Autodesk Inventor part; units mm, degrees
ref_plane "YZ Plane" through (0, 0, 0) normal (1, 0, 0) x (0, 1, 0)
ref_plane "XZ Plane" through (0, 0, 0) normal (0, 1, 0) x (-1, 0, 0)
ref_plane "XY Plane" through (0, 0, 0) normal (0, 0, 1) x (1, 0, 0)
sketch "Sketch1" plane through (0, 0, 0) normal (0, 0, 1) x (1, 0, 0)
  line L0 (0, 0) -> (112.522, 0)
  line L1 (112.522, 0) -> (112.522, 146.812)
  line L2 (112.522, 146.812) -> (0, 146.812)
  line L3 (0, 146.812) -> (0, 0)
  line L4 (7.62, 131.572) -> (104.902, 131.572)
  line L5 (104.902, 131.572) -> (104.902, 91.44)
  line L6 (104.902, 91.44) -> (7.62, 91.44)
  line L7 (7.62, 91.44) -> (7.62, 131.572)
  line L8 (21.59, 83.82) -> (90.932, 83.82)
  line L9 (90.932, 83.82) -> (90.932, 6.35)
  line L10 (90.932, 6.35) -> (21.59, 6.35)
  line L11 (21.59, 6.35) -> (21.59, 83.82)
  dimension "d0" = 97.282
  dimension "d1" = 40.132
  dimension "d2" = 69.342
  dimension "d3" = 77.47
  dimension "d4" = 6.35
  dimension "d5" = 21.59
  dimension "d6" = 7.62
  dimension "d7" = 7.62
  dimension "d8" = 15.24
  dimension "d9" = 7.62
extrude "Extrusion1" add sketch "Sketch1" along normal blind 9.4996 contours L3 L2 L1 L0 | L8 L9 L10 L11
sketch "Sketch2" plane through (0, 0, 9.4996) normal (0, 0, 1) x (1, 0, 0)
  line L0 (0, 0) -> (112.522, 0)
  line L1 (112.522, 0) -> (112.522, 139.192)
  line L2 (112.522, 139.192) -> (0, 139.192)
  line L3 (0, 139.192) -> (0, 0)
  line L4 (7.62, 131.572) -> (104.902, 131.572)
  line L5 (104.902, 131.572) -> (104.902, 91.44)
  line L6 (104.902, 91.44) -> (7.62, 91.44)
  line L7 (7.62, 91.44) -> (7.62, 131.572)
  line L8 (21.59, 83.82) -> (90.932, 83.82)
  line L9 (90.932, 83.82) -> (90.932, 6.35)
  line L10 (90.932, 6.35) -> (21.59, 6.35)
  line L11 (21.59, 6.35) -> (21.59, 83.82)
  line L12 (20.32, 85.09) -> (92.202, 85.09)
  line L13 (92.202, 85.09) -> (92.202, 5.08)
  line L14 (92.202, 5.08) -> (20.32, 5.08)
  line L15 (20.32, 5.08) -> (20.32, 85.09)
  dimension "d12" = 97.282
  dimension "d13" = 40.132
  dimension "d14" = 69.342
  dimension "d15" = 77.47
  dimension "d16" = 6.35
  dimension "d17" = 21.59
  dimension "d18" = 7.62
  dimension "d19" = 7.62
  dimension "d20" = 7.62
  dimension "d21" = 7.62
  dimension "d33" = 1.27
  dimension "d34" = 1.27
  dimension "d35" = 1.27
  dimension "d36" = 1.27
extrude "Extrusion2" cut sketch "Sketch2" against normal blind 0.0025 contours L12 L13 L14 L15
sketch "Sketch3" plane through (0, 0, 9.4996) normal (0, 0, 1) x (1, 0, 0)
  circle A0 centre (9.7155, 138.9888) radius 1.651
  circle A1 centre (102.7811, 138.9888) radius 1.651
  circle A2 centre (102.7811, 84.0232) radius 1.651
  circle A3 centre (9.7155, 84.0232) radius 1.651
  line L0 (104.902, 131.572) -> (104.902, 91.44)
  line L1 (104.902, 91.44) -> (7.62, 91.44)
  line L2 (21.59, 6.35) -> (90.932, 6.35)
  line L3 (92.202, 5.08) -> (20.32, 5.08)
  line L4 (46.101, 6.35) -> (66.421, 6.35)
  line L5 (66.421, 6.35) -> (66.421, 5.08)
  line L6 (66.421, 5.08) -> (46.101, 5.08)
  line L7 (46.101, 5.08) -> (46.101, 6.35)
  line L8 (21.59, 83.82) -> (21.59, 6.35)
  line L9 (90.932, 6.35) -> (90.932, 83.82)
  point P0 (0, 0)
  dimension "d24" = 3.302
  dimension "d25" = 93.0656
  dimension "d26" = 93.0656
  dimension "d27" = 0
  dimension "d28" = 54.9656
  dimension "d29" = 2.1209
  dimension "d30" = 0
  dimension "d31" = 7.4168
  dimension "d32" = 0
  dimension "d37" = 20.32
  dimension "d38" = 24.511
  dimension "d39" = 24.511
extrude "Extrusion3" cut sketch "Sketch3" against normal through all
sketch "Sketch10" plane through (0, 0, 0) normal (0, 0, -1) x (-1, 0, 0)
  line L0 (12.7738, 184.0109) -> (-117.8029, 184.0109)
  line L1 (-117.8029, 184.0109) -> (-117.8029, -18.4511)
  line L2 (-117.8029, -18.4511) -> (12.7738, -18.4511)
  line L3 (12.7738, -18.4511) -> (12.7738, 184.0109)
  line L4 (-5.08, 138.9888) -> (-5.08, 84.0232)
  line L5 (-14.351, 134.112) -> (-98.1202, 134.112)
  line L6 (-107.442, 138.9888) -> (-107.442, 84.0232)
  line L7 (-112.522, 0) -> (-112.522, 146.812)
  line L8 (-14.351, 88.9) -> (-98.1202, 88.9)
  arc A0 (-5.08, 138.9888) -> (-14.351, 138.9888) centre (-9.7155, 138.9888) ccw
  arc A1 (-14.351, 84.0232) -> (-5.08, 84.0232) centre (-9.7155, 84.0232) ccw
  arc A2 (-107.442, 84.0232) -> (-98.1202, 84.0232) centre (-102.7811, 84.0232) ccw
  arc A3 (-98.1202, 138.9888) -> (-107.442, 138.9888) centre (-102.7811, 138.9888) ccw
  circle A4 centre (-9.7155, 84.0232) radius 1.651
  circle A5 centre (-9.7155, 138.9888) radius 1.651
  circle A6 centre (-102.7811, 138.9888) radius 1.651
  circle A7 centre (-102.7811, 84.0232) radius 1.651
  line L9 (-14.351, 134.112) -> (-14.351, 138.9888)
  line L10 (-98.1202, 138.9888) -> (-98.1202, 134.112)
  line L11 (-7.62, 131.572) -> (-7.62, 91.44)
  line L12 (-7.62, 131.572) -> (-104.902, 131.572)
  line L13 (-7.62, 91.44) -> (-104.902, 91.44)
  line L14 (-104.902, 131.572) -> (-104.902, 91.44)
  line L15 (-98.1202, 84.0232) -> (-98.1202, 88.9)
  line L16 (-14.351, 88.9) -> (-14.351, 84.0232)
  line L17 (0, 76.2) -> (-112.5015, 3.0431)
  line L18 (-112.5015, 3.0431) -> (-112.522, 0)
  line L19 (-112.522, 0) -> (1.3847, 74.0706)
  line L20 (1.3847, 74.0706) -> (0, 76.2)
  line L21 (1.524, 2.54) -> (-112.522, 76.2)
  line L22 (-112.522, 76.2) -> (-114.4017, 74.3903)
  line L23 (-114.4017, 74.3903) -> (0.1459, 0.4063)
  line L24 (0.1459, 0.4063) -> (1.524, 2.54)
  line L25 (0, 0) -> (-112.522, 0)
  line L26 (0, 146.812) -> (0, 0)
  point P0 (-14.351, 136.5504)
  dimension "d64" = 2.54
  dimension "d65" = 2.54
  dimension "d66" = 2.54
  dimension "d67" = 2.54
  dimension "d68" = 2.54
  dimension "d69" = 2.54
  dimension "d70" = 2.54
  dimension "d71" = 1.524
  dimension "d72" = 76.2
  dimension "d73" = 0
  dimension "d74" = 76.2
  dimension "d75" = 0
  dimension "d76" = 0
  dimension "d77" = 0
extrude "Extrusion8" cut sketch "Sketch10" against normal blind 6.858 contours L3 L2 L1 L0 | L7 L23 L17 L18 | L19 L23 L26 L25 | L19 L26 L21
sketch "Sketch5" plane through (112.522, 0, 9.4996) normal (1, 0, 0) x (0, 0, -1)
  line L0 (9.4996, 146.812) -> (0, 146.812)
  line L1 (9.4996, 146.812) -> (75.9867, 115.8086)
  line L2 (9.4996, 0) -> (0, 0)
  line L3 (18.0577, -8.4205) -> (0, 0)
  line L4 (0, 146.812) -> (0, 0)
  line L5 (0, 0) -> (0, 146.812)
  line L6 (0, 146.812) -> (9.4996, 146.812)
  line L7 (75.9867, 115.8086) -> (18.0577, -8.4205)
  line L8 (22.86, 146.812) -> (22.86, 73.406)
  line L9 (9.4996, 0) -> (9.4996, 146.812)
  point P0 (5.08, 0)
  point P1 (9.4996, 80.01)
  point P2 (22.86, 80.01)
  dimension "d45" = 25
  dimension "d47" = 22.86
  dimension "d48" = 33.02
extrude "Extrusion5" add sketch "Sketch5" against normal blind 2.54
ref_plane "Work Plane1" through (56.261, 0, 9.4996) normal (-1, 0, 0) x (0, 0, 1)
mirror "Mirror1" about plane through (56.261, 0, 9.4996) normal (-1, 0, 0) of "Extrusion5"
sketch "Sketch7" plane through (112.522, 0, 9.4996) normal (1, 0, 0) x (0, 0, -1)
  line L0 (18.0577, -8.4205) -> (0, 0)
  line L1 (0, 0) -> (18.0577, -8.4205)
  line L2 (18.0577, -8.4205) -> (19.1312, -6.1184)
  line L3 (75.9867, 115.8086) -> (18.0577, -8.4205)
  line L4 (0, 2.8026) -> (0, 0)
  line L5 (0.0025, 6.35) -> (0.0025, 83.82)
  line L6 (19.1312, -6.1184) -> (0, 2.8026)
  line L7 (9.4996, 146.812) -> (0, 146.812)
  line L8 (9.4996, 146.812) -> (9.4996, 144.0094)
  line L9 (9.4996, 146.812) -> (9.4996, 0)
  line L10 (9.4996, 144.0094) -> (40.3829, 129.6083)
  line L11 (40.3829, 129.6083) -> (41.4564, 131.9103)
  line L12 (9.4996, 146.812) -> (75.9867, 115.8086)
  line L13 (41.4564, 131.9103) -> (9.4996, 146.812)
  line L14 (0, 146.812) -> (9.4996, 146.812)
  line L15 (9.4996, 144.0094) -> (0, 144.0094)
  line L16 (0, 146.812) -> (0, 0)
  line L17 (0, 144.0094) -> (0, 146.812)
  point P0 (9.4996, 80.01)
  point P1 (2.6416, 146.812)
  dimension "d51" = 2.54
  dimension "d61" = 2.54
  dimension "d63" = 38.1
extrude "Extrusion6" add sketch "Sketch7" against normal through all contours L0 L4 L6 L2 | L16 L7 L8 L15 | L11 L10 L8 L12
sketch "Sketch8" plane through (112.522, 0, 9.4996) normal (1, 0, 0) x (0, 0, -1)
  circle A0 centre (19.1087, 5.1024) radius 1.5875
  circle A1 centre (66.3031, 106.3112) radius 1.5875
  line L0 (0, 0) -> (18.0577, -8.4205)
  line L1 (18.0577, -8.4205) -> (75.9867, 115.8086)
  line L2 (75.9867, 115.8086) -> (9.4996, 146.812)
  point P0 (9.4996, 0)
  dimension "d54" = 3.175
  dimension "d55" = 12.7
  dimension "d56" = 4.7625
  dimension "d57" = 4.7625
  dimension "d80" = 12.7
extrude "Extrusion7" cut sketch "Sketch8" against normal through all
properties part number "face"
Source: CAD feature listing. Evaluate the final solid. Frame: model axes, mm. A direction names the side the tool comes from. Coordinates: 2 decimals unless noted, no trailing zeros. Loops run counter-clockwise (first coordinate to the right, second up) from the corner with the lowest first, then second, coordinate; pieces in that order, holes last. Notation, with made-up numbers: (-33.5, 18.25) - (-23.5, 18.25) arc R25 ccw to (-23.5, 34.25) - close; hole circle Ø3 at (-14, 59). An arc over 180 degrees is marked (long way). One line per item, written item: value. Start each with the question number.
1. Section A-A (z = -48.5). Return the cut outline in (x, y).
2. Mould query, pull axis Z, two halves, no side actions, for faces 1 (the flat face through (56, 134.112, 3)), 2 (the cylindrical face through (102.68, 143.65, 3.38)), 3 (the flat face through (112.522, 85, -21)). Classes: pulls with the +Z half, pulls with the -Z half, needs draft (parallel to the pull), parting line crosses it, or undercut.
3. Contact query for flat-ended pins moving along their axis: P1, Ø10.5, axis at x = 47, z = 3, coming from the -Y side; P2, Ø12, axis at x = 28, z = -1.5, coming from the -Y side; P3, Ø2, axis at x = 67, z = 2, coming from the -Y side. Output: stop coordinate, or through.
4. Set-up query: faces 4 (the flat face through (56, 131.572, 5)), 5 (the flat face through (83.401, 18.937, 3.381)), 6 (the flat face through (57, 144.009, 3)). Return all of +Z, -Z, +X, -X, +Y, -Y with unobstructed straight access to the full face (end or side cutting, diameter ignored); none if empty.
5. Ray query, L1, parallel to X at y = 89.5, z = -20; L2, parallel to Y at x = 86, z = 1; L3, parallel to Z at x = 49, y = 5. Return the intervals inside material, ascending.
6. Section D-D (x = 64). State how many separate pieces and enclosed holes the cut face has, and give its area (3 significant figures).
Verdict:
1. outline: (0, 77.24) - (2.54, 77.24) - (2.54, 124.2) - (0, 124.2) - close; (109.98, 77.24) - (112.52, 77.24) - (112.52, 124.2) - (109.98, 124.2) - close
2. face 1: undercut
2. face 2: undercut
2. face 3: needs draft
3. P1: stops at y = -5.48
3. P2: stops at y = -7.93
3. P3: stops at y = -3.96
4. face 4: +Z
4. face 5: -Z
4. face 6: none
5. L1: x = 0 to 2.54, 109.98 to 112.52
5. L2: y = -3.96 to -1.16, 17.25 to 20.28, 56.05 to 59.07, 88.9 to 91.44, 131.57 to 134.11, 144.01 to 146.81
5. L3: z = 6.86 to 9.5
6. separate pieces: 3
6. enclosed holes: 0
6. area: 508 mm2
